Check sheet for the modelled part. Datum: model origin and axes. Units: mm. Give positions to 0.01 mm unless a question says otherwise; leave off trailing zeros. Order: outer loops, then holes, each group sorted by start corner. A loop starts at its lowest first (then second) coordinate and runs counter-clockwise, first axis right, second up.
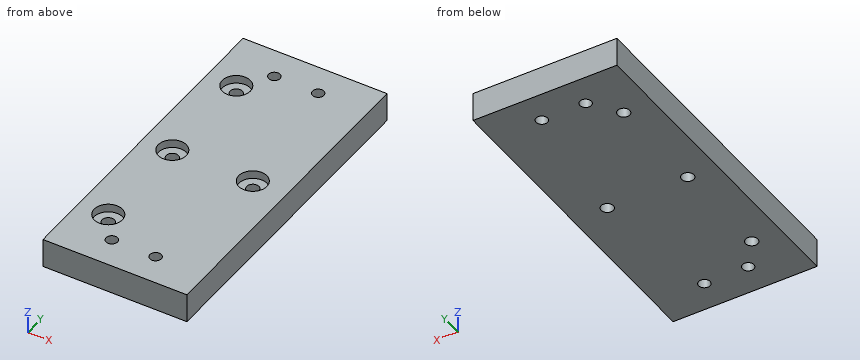
Autodesk Inventor part; units mm, degrees
ref_plane "YZ Plane" through (0, 0, 0) normal (1, 0, 0) x (0, 1, 0)
ref_plane "XZ Plane" through (0, 0, 0) normal (0, 1, 0) x (-1, 0, 0)
ref_plane "XY Plane" through (0, 0, 0) normal (0, 0, 1) x (1, 0, 0)
sketch "Sketch1" plane through (0, 0, 0) normal (0, 0, 1) x (1, 0, 0)
  line L0 (0, 0) -> (62.5348, 0)
  line L1 (62.5348, 0) -> (62.5348, 140.716)
  line L2 (62.5348, 140.716) -> (0, 140.716)
  line L3 (0, 140.716) -> (0, 0)
  line L4 (0, 70.358) -> (62.5348, 70.358)
  circle A0 centre (12.7, 70.358) radius 2.5
  circle A1 centre (12.7, 115.358) radius 2.5
  circle A2 centre (12.7, 25.358) radius 2.5
  circle A3 centre (21.7424, 127.508) radius 3.175
  circle A4 centre (21.7424, 13.208) radius 3.175
  circle A5 centre (40.7924, 127.508) radius 3.175
  circle A6 centre (40.7924, 13.208) radius 3.175
  circle A7 centre (47.7, 70.358) radius 2.5
  dimension "d0" = 140.716
  dimension "d1" = 5
  dimension "d2" = 12.7
  dimension "d3" = 45
  dimension "d5" = 6.35
  dimension "d6" = 114.3
  dimension "d10" = 19.05
  dimension "d16" = 35
  dimension "d33" = 62.5348
  dimension "d34" = 21.7424
  dimension "d35" = 21.7424
extrude "Extrusion1" add sketch "Sketch1" against normal blind 12.7 contours L3 L4 A0 A7 L1 L0 | L3 L2 L1 L4 A7 A0 | A0 L4 | L4 A0 | A7 L4 | L4 A7 | A1 | A2 | A3 | A4 | A5 | A6
hole "Hole1" at (12.7, 115.358, 0) at (12.7, 70.358, 0) at (12.7, 25.358, 0) at (47.7, 70.358, 0) direction (0, 0, -1) diameter 5.3086 end through all counterbore diameter 12.2428 counterbore depth 3.5814
hole "Hole2" at (21.7424, 13.208, 0) at (40.7924, 13.208, 0) at (40.7924, 127.508, 0) at (21.7424, 127.508, 0) direction (0, 0, -1) diameter 4.9784 end through all
equation "\"d34\" = d35"
properties part number "Fixed Side Adapter Plate"
1) Section check A-A, the plane x = 12.7. Record the cut outline in (y, z).
Recorded:
outline: (0, -12.7) - (22.7, -12.7) - (22.7, -3.58) - (19.24, -3.58) - (19.24, 0) - (0, 0) - close; (28.01, -12.7) - (67.7, -12.7) - (67.7, -3.58) - (64.24, -3.58) - (64.24, 0) - (31.48, 0) - (31.48, -3.58) - (28.01, -3.58) - close; (73.01, -12.7) - (112.7, -12.7) - (112.7, -3.58) - (109.24, -3.58) - (109.24, 0) - (76.48, 0) - (76.48, -3.58) - (73.01, -3.58) - close; (118.01, -12.7) - (140.72, -12.7) - (140.72, 0) - (121.48, 0) - (121.48, -3.58) - (118.01, -3.58) - close
2) Section check B-B, the plane z = -1.5. State how many separate pieces and enclosed holes the cut face has, then the cut area to 3 significant figures.
Recorded:
separate pieces: 1
enclosed holes: 8
area: 8,250 mm2
3) Depth check by flat-ended pin: pin 1 Ø8.5 at (x, y) = (12.7, 70.358) entering from +Z; pin 2 Ø3 at (y, z) = (31.5, -9) entering from -X; pin 3 Ø4.5 at (x, y) = (40.79, 127.51) entering from -Z. Enter the tip coordinate at first touch or a pass-through.
Recorded:
pin 1: stops at z = -3.58
pin 2: stops at x = 0
pin 3: passes through
4) Material ranges on L1, parallel to Y at x = 12.7, z = -0.7; L2, parallel to Y at x = 21.5, z = -11.75; L3, parallel to Y at x = 11, z = -6.25, recorded low to high.
Recorded:
L1: y = 0 to 19.24, 31.48 to 64.24, 76.48 to 109.24, 121.48 to 140.72
L2: y = 0 to 10.73, 15.69 to 125.03, 129.99 to 140.72
L3: y = 0 to 23.32, 27.4 to 68.32, 72.4 to 113.32, 117.4 to 140.72
5) Section check C-C, the plane x = 47.7. Record the cut outline in (y, z).
Recorded:
outline: (0, -12.7) - (67.7, -12.7) - (67.7, -3.58) - (64.24, -3.58) - (64.24, 0) - (0, 0) - close; (73.01, -12.7) - (140.72, -12.7) - (140.72, 0) - (76.48, 0) - (76.48, -3.58) - (73.01, -3.58) - close
